The figure shows three views and two pictorial views of one solid part (mm, origin at its lowest corner). Answer the questions. A direction names the side the tool comes from. Coordinates: 2 decimals unless noted, no trailing zeros. Loops run counter-clockwise (first coordinate to the right, second up) from the corner with the lowest first, then second, coordinate; pieces in that order, holes last. Notation, with made-up numbers: (17.5, 5) - (29.5, 5) arc R31 ccw to (29.5, 30) - close; hole circle Ø3 at (1, 71). An arc over 180 degrees is marked (long way). Return JSON: item names as keys, results as strings. Group by question number.
1. Find the intervals of material crossed by line 1 along Z through (x, y) = (46.5, 551); line 2 along X through (y, z) = (393.5, 1129); line 3 along X through (y, z) = (404.5, 662), in increasing order.
2. Each of these flat-tipped pins is pushed along its axis until it touches: P1, Ø6, axis at x = 259, y = 95, coming from the -Z side; P2, Ø2, axis at x = 380.5, z = 298.5, coming from the +Y side. Where does it stop, or does it pass through?
3. Section C-C (z = 169.5) is taken. Write down the section's boundary in (x, y).
4. Section D-D (x = 233.5) is taken. Write down the section's boundary in (y, z), and give its area (3 significant figures).
5. Section A-A (y = 400) is taken. Write down the section's boundary in (x, z).
6. Which of the six approach directions +Z, -Z, +X, -X, +Y, -Y give full straight-line access (tool end or side, diameter ignored) to the marked faces 1 and 2?
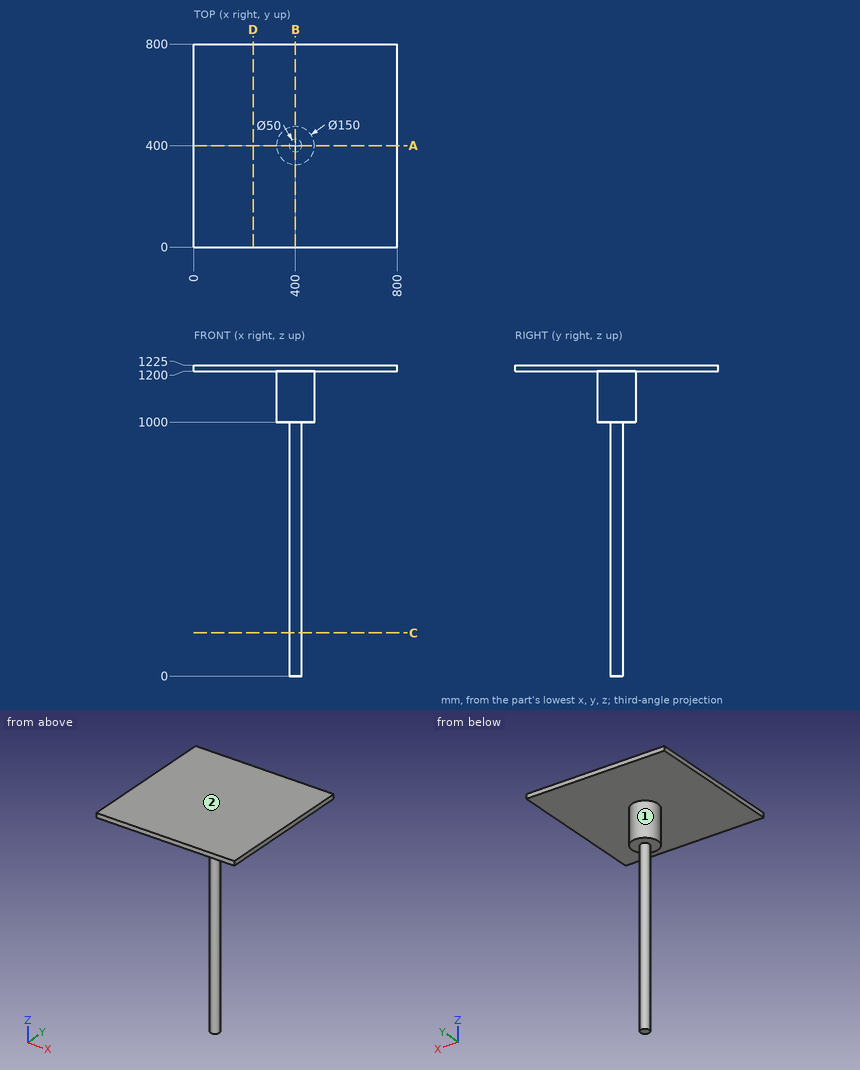
The answers:
{
 "1": {"line 1": "z = 1200 to 1225", "line 2": "x = 325.28 to 474.72", "line 3": "x = 375.41 to 424.59"},
 "2": {"P1": "stops at z = 1200", "P2": "stops at y = 416.82"},
 "3": {"outline": "circle Ø50 at (400, 400)"},
 "4": {"outline": "(0, 1200) - (800, 1200) - (800, 1225) - (0, 1225) - close", "area": "20,000 mm2"},
 "5": {"outline": "(0, 1200) - (325, 1200) - (325, 1000) - (375, 1000) - (375, 0) - (425, 0) - (425, 1000) - (475, 1000) - (475, 1200) - (800, 1200) - (800, 1225) - (0, 1225) - close"},
 "6": {"face 1": "-Z", "face 2": "+Z, +X, -X, +Y, -Y"}
}
